from build123d import *

# Parameters (mm, degrees)
BOSS_EXTRUDE4_DEPTH = 40
SKETCH5_R           = 10.720024077
CUT_EXTRUDE1_DEPTH  = 120


with BuildPart() as part:
    # Sketch1 → Boss-Extrude4 (new body)
    with BuildSketch(Plane(origin=(0, 0, 0), x_dir=(1, 0, 0), z_dir=(0, 1, 0))):
        Polygon((-101.900826446, 53.429752066), (-101.900826446, -96.570247934), (18.099173554, -96.570247934), (18.099173554, 53.429752066), (-21.900826446, 103.429752066), (-41.900826446, 103.429752066), (-61.900826446, 103.429752066), align=None)
    extrude(amount=BOSS_EXTRUDE4_DEPTH)

    # Sketch5 → Cut-Extrude1 (cut)
    with BuildSketch(Plane.ZY.offset(101.900826446)):
        with Locations((71.572647324, 20.323286204)):
            Circle(SKETCH5_R)
    extrude(amount=-CUT_EXTRUDE1_DEPTH, mode=Mode.SUBTRACT)


solid = part.part
Design review of the part built by this model. Coordinates are the model's own, in mm. Give positions to 0.01 mm unless a question says otherwise; leave off trailing zeros. Loops run counter-clockwise (first coordinate to the right, second up) from the corner with the lowest first, then second, coordinate; pieces in that order, holes last. Notation, with made-up numbers: M 61.5,-26 L 100.5,-26 A15 ccw 100.5,-10 Z; hole C -14,66.25 d7. An arc over 180 degrees is marked long. Answer as a JSON object with one key per item and string values.
Item 1: For P1, Ø5, axis at x = -80, y = 10, coming from the -Z side; P2, Ø2, axis at y = 10.5, z = -82.5, coming from the -X side; P3, Ø8, axis at y = 35, z = -76, coming from the -X side, all flat-tipped, find the tip position at first contact; note any pin that passes through.
Output values:
{"P1": "stops at z = -83.93", "P2": "stops at x = -79.44", "P3": "stops at x = -87.04"}
Item 2: Mouldability with a two-part tool opening along Z and no side actions: class faces 1 (the face through (-42, 20, -103.43)), 2 (the face through (-42.741, 20.795, 60.863)), 3 (the face through (-43, 20, 96.57)) as pulls with the +Z half, pulls with the -Z half, needs draft (parallel to the pull), parting line crosses it, or undercut.
Output values:
{"face 1": "pulls with the -Z half", "face 2": "undercut", "face 3": "pulls with the +Z half"}
Item 3: Wall thickness on line 1 along Z through (x, y) = (-42, 20.5); line 2 along Z through (x, y) = (-49.5, 18); line 3 along Y through (x, z) = (-95.5, 74.5): over which ranges is each line inside the solid? List them lowest first.
Output values:
{"line 1": "z = -103.43 to 60.85, 82.29 to 96.57", "line 2": "z = -103.43 to 61.11, 82.04 to 96.57", "line 3": "y = 0 to 10.01, 30.64 to 40"}
Item 4: We need section A-A (y = 23.5). State the section outline as (x, z) points.
Output values:
{"outline": "M -101.9,-53.43 L -61.9,-103.43 L -21.9,-103.43 L 18.1,-53.43 L 18.1,61.33 L -101.9,61.33 Z; M -101.9,81.81 L 18.1,81.81 L 18.1,96.57 L -101.9,96.57 Z"}
Item 5: We need section D-D (y = 14). State the section outline as (x, z) points, and give its area (3 significant figures).
Output values:
{"outline": "M -101.9,-53.43 L -61.9,-103.43 L -21.9,-103.43 L 18.1,-53.43 L 18.1,62.92 L -101.9,62.92 Z; M -101.9,80.23 L 18.1,80.23 L 18.1,96.57 L -101.9,96.57 Z", "area": "19,900 mm2"}
Item 6: We need section C-C (y = 35). State the section outline as (x, z) points, and give its area (3 significant figures).
Output values:
{"outline": "M -101.9,-53.43 L -61.9,-103.43 L -21.9,-103.43 L 18.1,-53.43 L 18.1,96.57 L -101.9,96.57 Z", "area": "22,000 mm2"}
Item 7: We need section B-B (x = -5). State the section outline as (y, z) points.
Output values:
{"outline": "M 0,-82.3 L 40,-82.3 L 40,96.57 L 0,96.57 Z; hole C 20.32,71.57 d21.44"}
